Could you check a few things on this drawing? It's one solid part, dimensions in mm from its lowest x, y, z. Give positions to 0.01 mm unless a question says otherwise; leave off trailing zeros. Order: outer loops, then holes, each group sorted by start corner. A loop starts at its lowest first (then second) coordinate and runs counter-clockwise, first axis right, second up.
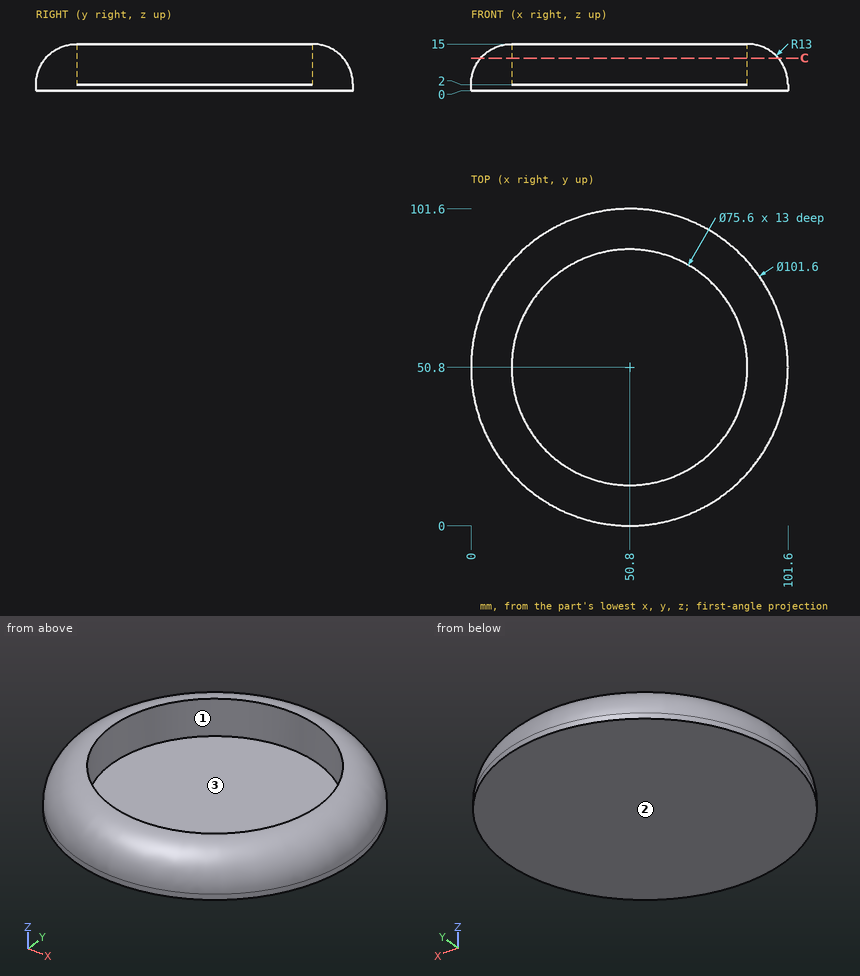
Item 1: We'd pull the mould along Y, two halves only. Please class the marked faces 1, 2 and 3: +Y half, -Y half, draft (parallel to the pull), parting line (faces both ways), or undercut.
Findings:
face 1: undercut
face 2: draft
face 3: undercut
Item 2: For pin 1 (4 mm diameter, centred on y = 30.5, z = 12.5, fed in from -X); pin 2 (3 mm diameter, centred on x = 67.5, z = 10, fed in from +Y); pin 3 (22.5 mm diameter, centred on x = 63.5, y = 46, fed in from +Z), each with a flat end and sliding along its axis, tell me the tip position at first contact or that it passes through.
Findings:
pin 1: stops at x = 7.5
pin 2: stops at y = 97.07
pin 3: stops at z = 2
Item 3: Please list where these lines run through material, in increasing order: line 1 along Z through (x, y) = (23, 58); line 2 along Y through (x, z) = (64, 2.25); line 3 along Y through (x, z) = (65.5, 6.5).
Findings:
line 1: z = 0 to 2
line 2: y = 1.75 to 15.38, 86.22 to 99.85
line 3: y = 3.01 to 15.98, 85.62 to 98.59
Item 4: Imagine slicing it at C-C on z = 10.5. List the corners of the cut face in (x, y) for me, then the cut area to 3 significant figures.
Findings:
outline: circle Ø95.27 at (50.8, 50.8); hole circle Ø75.6 at (50.8, 50.8)
area: 2,640 mm2
